```python
from build123d import *

# Parameters (mm, degrees)
ESQUISSE1_R        = 2.25
BOSS_EXTRU_1_DEPTH = 4
CONG_2_R           = 6
CONG_3_R           = 20
ESQUISSE2_R        = 10.75
BOSS_EXTRU_2_DEPTH = 4.5


with BuildPart() as part:
    # Esquisse1 → Boss.-Extru.1 (new body)
    with BuildSketch(Plane.XY):
        Polygon((-55, 20), (-27.5, 0), (0, 20), (0, 40), (-55, 40), align=None)
        with Locations((-47.5, 32.5)):
            Circle(ESQUISSE1_R, mode=Mode.SUBTRACT)
        with Locations((-7.5, 32.5)):
            Circle(ESQUISSE1_R, mode=Mode.SUBTRACT)
        with Locations((-27.5, 7.5)):
            Circle(ESQUISSE1_R, mode=Mode.SUBTRACT)
    extrude(amount=BOSS_EXTRU_1_DEPTH)

    # Congé2
    cong_2_edges = [part.edges().sort_by_distance(p)[0] for p in [
        (-55, 40, 2),
        (0, 40, 2),
        (-27.5, 0, 2),
    ]]
    fillet(cong_2_edges, radius=CONG_2_R)

    # Congé3
    cong_3_edges = [part.edges().sort_by_distance(p)[0] for p in [
        (0, 20, 2),
        (-55, 20, 2),
    ]]
    fillet(cong_3_edges, radius=CONG_3_R)

    # Esquisse2 → Boss.-Extru.2 (add)
    with BuildSketch(Plane(origin=(0, 0, 0), x_dir=(-1, 0, 0), z_dir=(0, 0, -1))):
        with Locations(Location((27.5, 27.5, 0), (0, 0, 180))):  # turned: the seam where the file's is
            Circle(ESQUISSE2_R)
    extrude(amount=BOSS_EXTRU_2_DEPTH)


solid = part.part
```
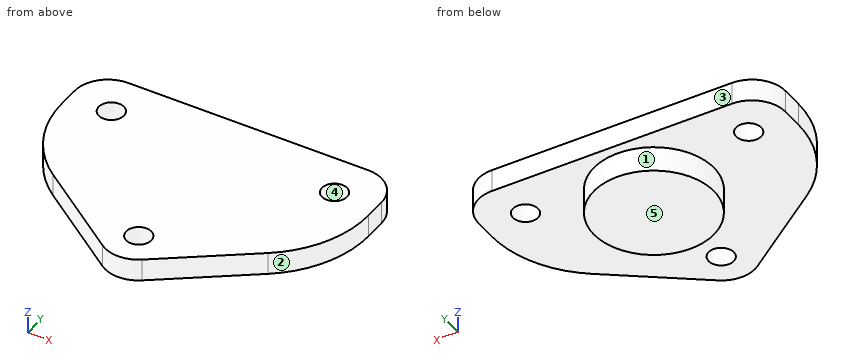
Input: part model. Units: mm. Frame: model coordinates. Face numbers are marked on the shaded views. A direction names the side the tool comes from. Round coordinates to 2 decimals unless told otherwise and drop trailing zeros. Order: outer loops, then holes, each group sorted by start corner. A loop starts at its lowest first (then second) coordinate and runs counter-clockwise, first axis right, second up. Notation, with made-up numbers: (76, 33.5) - (109, 33.5) arc R33 ccw to (109, 66.5) - close; hole circle Ø9 at (-25.75, 29). An arc over 180 degrees is marked (long way). Answer in a Markdown table with one row per item.
Item 1: Reachability of the marked faces 1 and 2 from +Z, -Z, +X, -X, +Y, -Y: full face, straight path, thin tool, end or side. Return the list, or none.
Model answer:
| item | result |
|---|---|
| face 1 | -Z |
| face 2 | +Z, -Z, +X, -Y |
Item 2: Mould query, pull axis Y, two halves, no side actions, for the marked faces 3, 4 and 5. Classes: released by +Y, released by -Y, zero draft, split by the parting line, or undercut.
Model answer:
| item | result |
|---|---|
| face 3 | released by +Y |
| face 4 | undercut |
| face 5 | zero draft |
Item 3: Pin query (flat end, axial travel): pin 1 (4 mm diameter, centred on y = 18.5, z = 0, fed in from +X); pin 2 (3 mm diameter, centred on x = -11.5, z = 2, fed in from -Y); pin 3 (4 mm diameter, centred on x = -19.5, z = -0.5, fed in from -Y); pin 4 (1.5 mm diameter, centred on x = -28, y = 8.5, fed in from +Z). Return the tip coordinate at first contact, or that it passes through.
Model answer:
| item | result |
|---|---|
| pin 1 | stops at x = -2.5 |
| pin 2 | stops at y = 10.55 |
| pin 3 | stops at y = 4.41 |
| pin 4 | passes through |
Item 4: Line query: line 1 (Y direction, x = -27.5, z = 3); line 2 (Z direction, x = -9, y = 15); line 3 (Y direction, x = -47, z = 2.5). Output: solid intervals per line, ascending.
Model answer:
| item | result |
|---|---|
| line 1 | y = 1.42 to 5.25, 9.75 to 40 |
| line 2 | z = 0 to 4 |
| line 3 | y = 14.18 to 30.31, 34.69 to 40 |
Item 5: Section query B-B (x = -27.5). Return the cut outline in (y, z), then the cut area to 3 significant figures.
Model answer:
| item | result |
|---|---|
| outline | (1.42, 0) - (5.25, 0) - (5.25, 4) - (1.42, 4) - close; (9.75, 0) - (16.75, 0) - (16.75, -4.5) - (38.25, -4.5) - (38.25, 0) - (40, 0) - (40, 4) - (9.75, 4) - close |
| area | 233 mm² |
Item 6: Section query A-A (y = 32.5). Return the cut outline in (x, z).
Model answer:
| item | result |
|---|---|
| outline | (-55, 0) - (-49.75, 0) - (-49.75, 4) - (-55, 4) - close; (-45.25, 0) - (-37.02, 0) - (-37.02, -4.5) - (-17.98, -4.5) - (-17.98, 0) - (-9.75, 0) - (-9.75, 4) - (-45.25, 4) - close; (-5.25, 0) - (0, 0) - (0, 4) - (-5.25, 4) - close |
Item 7: Section query C-C (y = 6.5). Return the cut outline in (x, z).
Model answer:
| item | result |
|---|---|
| outline | (-36.44, 0) - (-29.52, 0) - (-29.52, 4) - (-36.44, 4) - close; (-25.48, 0) - (-18.56, 0) - (-18.56, 4) - (-25.48, 4) - close |
Item 8: Section query D-D (x = -36). Return the cut outline in (y, z).
Model answer:
| item | result |
|---|---|
| outline | (6.18, 0) - (20.92, 0) - (20.92, -4.5) - (34.08, -4.5) - (34.08, 0) - (40, 0) - (40, 4) - (6.18, 4) - close |
